```python
from build123d import *

# Parameters (mm, degrees)
F1_DEPTH = 25.4
F2_R     = 6.35
F3_DEPTH = 12.701
F5_DEPTH = 12.701
F7_DEPTH = 12.701


with BuildPart() as f1:
    # F0 (on Front) → F1 (new body)
    with BuildSketch(Plane.XZ):
        Polygon((-45.6721438388, 52.0613446782), (-58.3721438388, 52.0613446782), (-58.3721438388, 7.6113446782), (-1.2221438388, 7.6113446782), (-1.2221438388, 20.3113446782), (-45.6721438388, 20.3113446782), align=None)
    extrude(amount=F1_DEPTH)

    # F2 (on face) → F3 (cut, through all)
    with BuildSketch(Plane.XY.offset(20.3113446782)):
        with Locations((-32.9721438388, -12.7)):
            Circle(F2_R)
        with Locations((-13.9221438388, -12.7)):
            Circle(F2_R)
    extrude(amount=-F3_DEPTH, mode=Mode.SUBTRACT)

    # F4 (on face) → F5 (cut, through all)
    with BuildSketch(Plane.XY.offset(20.3113446782)):
        with BuildLine():
            ThreePointArc((-13.3388349786, 0), (-5.2890481293, -3.2694333282), (-1.2221438388, -10.9472293725))
            Line((-1.2221438388, -10.9472293725), (-1.2221438388, 0))
            Line((-1.2221438388, 0), (-13.3388349786, 0))
        make_face()
        with BuildLine():
            ThreePointArc((-1.2221438388, -14.447602267), (-5.3529503077, -22.1827419169), (-13.5104743141, -25.4))
            Line((-13.5104743141, -25.4), (-1.2221438388, -25.4))
            Line((-1.2221438388, -25.4), (-1.2221438388, -14.447602267))
        make_face()
    extrude(amount=-F5_DEPTH, mode=Mode.SUBTRACT)

    # F6 (on face) → F7 (cut, through all)
    with BuildSketch(Plane.YZ.offset(-45.6721438388)):
        with BuildLine():
            Line((-7.4811726809, 39.4210381167), (-7.4811726809, 50.9207851655))
            ThreePointArc((-7.4811726809, 50.9207851655), (-12.8712353004, 52.0348936879), (-18.2387330395, 50.8167061557))
            Line((-18.2387330395, 50.8167061557), (-18.2387330395, 39.0471868407))
            Line((-18.2387330395, 39.0471868407), (-18.0232445354, 39.0471868407))
            ThreePointArc((-18.0232445354, 39.0471868407), (-12.9326228444, 44.3215361788), (-7.4811726809, 39.4210381167))
        make_face()
        with BuildLine():
            ThreePointArc((-7.4811726809, 50.9207851655), (-2.5937691395, 47.1488570851), (0, 41.5464900434))
            Line((0, 41.5464900434), (0, 52.0613446782))
            Line((0, 52.0613446782), (-25.4, 52.0613446782))
            Line((-25.4, 52.0613446782), (-25.4, 41.9732704759))
            ThreePointArc((-25.4, 41.9732704759), (-22.839399389, 47.2209939486), (-18.2387330395, 50.8167061557))
            ThreePointArc((-18.2387330395, 50.8167061557), (-12.8712353004, 52.0348936879), (-7.4811726809, 50.9207851655))
        make_face()
        with BuildLine():
            Line((-7.4811726809, 39.0471868407), (-7.4811726809, 39.4210381167))
            ThreePointArc((-7.4811726809, 39.4210381167), (-12.9326228444, 44.3215361788), (-18.0232445354, 39.0471868407))
            Line((-18.0232445354, 39.0471868407), (-7.4811726809, 39.0471868407))
        make_face()
        with BuildLine():
            ThreePointArc((-7.4679148717, 39.0471868407), (-7.4712303654, 39.2342299815), (-7.4811726809, 39.4210381167))
            Line((-7.4811726809, 39.4210381167), (-7.4811726809, 39.0471868407))
            Line((-7.4811726809, 39.0471868407), (-18.0232445354, 39.0471868407))
            ThreePointArc((-18.0232445354, 39.0471868407), (-12.7455797036, 33.7695220088), (-7.4679148717, 39.0471868407))
        make_face()
    extrude(amount=-F7_DEPTH, mode=Mode.SUBTRACT)


solid = f1.part
```
The model under review builds one solid part; all positions refer to its coordinate system, in mm. A direction names the side the tool comes from. Give positions to 0.01 mm unless a question says otherwise; leave off trailing zeros. Write each loop counter-clockwise with the first axis right and the second up, starting at its lowest first coordinate (ties: lowest second). Pieces come first, ordered by that corner, then holes. Notation, with made-up numbers: (29, 32.5) -> (82, 32.5) arc R28 cw to (82, 62.5) -> close; hole circle Ø2 at (9, 84.25). An arc over 180 degrees is marked (long way). Put each result on its own line as item: value.
(1) We need section A-A, the plane z = 40.5. Give the boundary of the cut face in (x, y), and give its area (3 significant figures).
Results are:
outline: (-58.37, -25.4) -> (-45.67, -25.4) -> (-45.67, -18.24) -> (-58.37, -18.24) -> close; (-58.37, -7.48) -> (-45.67, -7.48) -> (-45.67, 0) -> (-58.37, 0) -> close
area: 186 mm²
(2) Tool access review of faces 5 (the flat face through (-23, -13, 20.311)), 6 (the flat face through (-52, -7.481, 45)), 7 (the cylindrical face through (-5.26, -22.1, 14.05)): name each direction out of +Z, -Z, +X, -X, +Y, -Y from which nothing blocks a thin tool from reaching the whole face with its end or side.
Results are:
face 5: +Z, +X, +Y, -Y
face 6: +Z, +X, -X
face 7: +Z, -Z, +X, -Y
(3) To check wall thickness, follow probe 1 along Z at (x, y) = (-41, -6); probe 2 along Y at (x, z) = (-48.5, 36); probe 3 along X at (y, z) = (-10.25, 20). State the ranges of each line that lie inside material, in increasing order. Write a range as from..to.
Results are:
probe 1: 7.61..20.31
probe 2: -25.4..-17.05, -8.44..0
probe 3: -58.37..-38.83, -27.11..-19.78, -8.06..-1.34
(4) For pin 1 Ø7.5 at (x, y) = (-16.5, -17) entering from +Z; pin 2 Ø4 at (y, z) = (-3, 18.5) entering from +X, all flat-tipped, find the tip position at first contact; note any pin that passes through.
Results are:
pin 1: z = 20.31
pin 2: x = -3.7
(5) We need section B-B, the plane z = 15. Give the boundary of the cut face in (x, y), and give its area (3 significant figures).
Results are:
outline: (-58.37, -25.4) -> (-13.51, -25.4) arc R12.71 ccw to (-1.22, -14.45) -> (-1.22, -10.95) arc R12.71 ccw to (-13.34, 0) -> (-58.37, 0) -> close; hole circle Ø12.7 at (-32.97, -12.7); hole circle Ø12.7 at (-13.92, -12.7)
area: 1,130 mm²
(6) We need section D-D, the plane x = -40. Give the boundary of the cut face in (y, z).
Results are:
outline: (-25.4, 7.61) -> (0, 7.61) -> (0, 20.31) -> (-25.4, 20.31) -> close
(7) We need section C-C, the plane y = -12.7. Give the boundary of the cut face in (x, z), and give its area (3 significant figures).
Results are:
outline: (-58.37, 7.61) -> (-39.32, 7.61) -> (-39.32, 20.31) -> (-45.67, 20.31) -> (-45.67, 33.77) -> (-58.37, 33.77) -> close; (-26.62, 7.61) -> (-20.27, 7.61) -> (-20.27, 20.31) -> (-26.62, 20.31) -> close; (-7.57, 7.61) -> (-1.22, 7.61) -> (-1.22, 20.31) -> (-7.57, 20.31) -> close
area: 574 mm²
(8) The part is to be moulded in two halves that separate along X. For faces 1 (the cylindrical face through (-18.961, -16.564, 14.05)), 2 (the flat face through (-41, 0, 17)), 3 (the cylindrical face through (-38.011, -16.564, 14.05)), 4 (the flat face through (-45.672, -13, 32)), say which applies: pulls with the +X half, pulls with the -X half, needs draft (parallel to the pull), parting line crosses it, or undercut.
Results are:
face 1: undercut
face 2: needs draft
face 3: undercut
face 4: pulls with the +X half
